from build123d import *

# Parameters (mm, degrees)
F4_R     = 1.5
F5_DEPTH = 12.5


with BuildPart() as f1:
    # F0 (on Top) → F1 (revolve)
    with BuildSketch(Plane.XY):
        Polygon((1.5, 3.5), (1.5, 0), (5.5, 0), (5.5, 3.5), (5.5, 6.5), (5.5, 10), (1.5, 10), (1.5, 6.5), align=None)
    revolve(axis=Axis((0, 15, 0), (0, -1, 0)))

    # F4 (on Right) → F5 (cut, symmetric)
    with BuildSketch(Plane.YZ):
        with Locations((5, 0)):
            Circle(F4_R)
    extrude(amount=F5_DEPTH, both=True, mode=Mode.SUBTRACT)


solid = f1.part
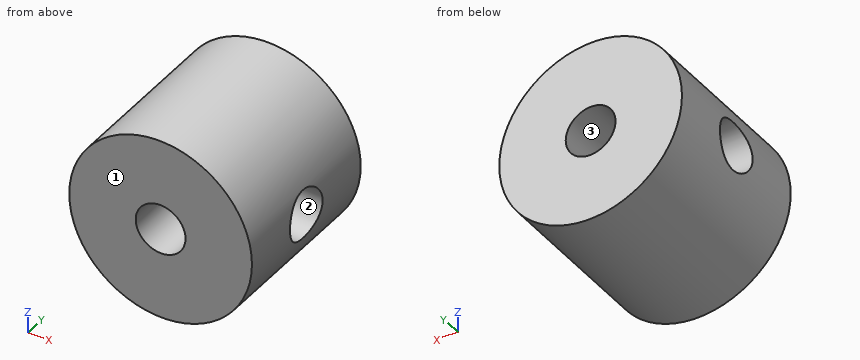
The model under review builds one solid part; all positions refer to its coordinate system, in mm. Face numbers are marked on the shaded views. Round coordinates to 2 decimals unless told otherwise and drop trailing zeros. Write each loop counter-clockwise with the first axis right and the second up, starting at its lowest first coordinate (ties: lowest second). Pieces come first, ordered by that corner, then holes. Notation, with made-up numbers: M -36.75,68 L 15.25,68 A17 cw 15.25,87 Z; hole C -3.5,17 d10. An arc over 180 degrees is marked long. Use a Markdown table: item, result. Add a question column.
Q1. We need section B-B, the plane y = 6. State the section outline as (x, z) points, plus the area to 3 significant figures.
Q2. We need section A-A, the plane z = 0. State the section outline as (x, y) points, plus the area to 3 significant figures.
Q3. Insertion check: pin 1 (3.5 mm diameter, centred on x = 0, z = 0, fed in from -Y); pin 2 (1.5 mm diameter, centred on x = -2.5, y = 2, fed in from -Z). Each pin has a flat end and moves straight along its axis. Give the tip position at first contact, or say it passes through.
Q4. To check wall thickness, follow line 1 (Z direction, x = 0, y = 8.35); line 2 (Y direction, x = 2.1, z = 0). State the ranges of each line that lie inside material, in increasing order.
Q5. We need section C-C, the plane x = -0.5. State the section outline as (y, z) points, plus the area to 3 significant figures.
Q6. The part is to be moulded in two halves that separate along Y. For the marked faces 1, 2 and 3, say which applies: pulls with the +Y half, pulls with the -Y half, needs draft (parallel to the pull), parting line crosses it, or undercut.
Q7. We need section D-D, the plane x = -3.5. State the section outline as (y, z) points.
Findings below:
| question | item | result |
|---|---|---|
| 1 | outline | M -5.39,-1.12 A5.5 ccw 5.39,-1.12 L 1,-1.12 A1.5 cw -1,-1.12 Z; M -5.39,1.12 L -1,1.12 A1.5 cw 1,1.12 L 5.39,1.12 A5.5 ccw Z |
| 1 | area | 69.6 mm² |
| 2 | outline | M -5.5,0 L -1.5,0 L -1.5,3.5 L -5.5,3.5 Z; M -5.5,6.5 L -1.5,6.5 L -1.5,10 L -5.5,10 Z; M 1.5,0 L 5.5,0 L 5.5,3.5 L 1.5,3.5 Z; M 1.5,6.5 L 5.5,6.5 L 5.5,10 L 1.5,10 Z |
| 2 | area | 56.0 mm² |
| 3 | pin 1 | stops at y = 0 |
| 3 | pin 2 | stops at z = -5.21 |
| 4 | line 1 | z = -5.5 to -1.5, 1.5 to 5.5 |
| 4 | line 2 | y = 0 to 3.5, 6.5 to 10 |
| 5 | outline | M 0,-5.48 L 10,-5.48 L 10,-1.41 L 5.5,-1.41 A1.5 cw 4.5,-1.41 L 0,-1.41 Z; M 0,1.41 L 4.5,1.41 A1.5 cw 5.5,1.41 L 10,1.41 L 10,5.48 L 0,5.48 Z |
| 5 | area | 81.1 mm² |
| 6 | face 1 | pulls with the -Y half |
| 6 | face 2 | undercut |
| 6 | face 3 | needs draft |
| 7 | outline | M 0,-4.24 L 10,-4.24 L 10,4.24 L 0,4.24 Z; hole C 5,0 d3 |
